Autodesk Inventor part; units mm, degrees
ref_plane "YZ Plane" through (0, 0, 0) normal (1, 0, 0) x (0, 1, 0)
ref_plane "XZ Plane" through (0, 0, 0) normal (0, 1, 0) x (-1, 0, 0)
ref_plane "XY Plane" through (0, 0, 0) normal (0, 0, 1) x (1, 0, 0)
sketch "스케치1" plane through (0, 0, 0) normal (0, 0, 1) x (1, 0, 0)
  circle A0 centre (0, 0) radius 2.5
  dimension "d0" = 5
extrude "돌출1" add sketch "스케치1" along normal mid plane 27
sketch "스케치2" plane through (0, 0, 13.5) normal (0, 0, 1) x (1, 0, 0)
  circle A0 centre (0, 0) radius 5
  dimension "d3" = 10
extrude "돌출2" add sketch "스케치2" along normal blind 3.5
sketch "스케치3" plane through (0, 0, -13.5) normal (0, 0, -1) x (-1, 0, 0)
  circle A0 centre (0, 0) radius 5
  dimension "d6" = 10
extrude "돌출3" add sketch "스케치3" along normal blind 3.5
sketch "스케치4" plane through (0, 0, 0) normal (0, 1, 0) x (-1, 0, 0)
  line L0 (-2, 3) -> (2, 3)
  line L1 (2, 3) -> (2, -3)
  line L2 (2, -3) -> (-2, -3)
  line L3 (-2, -3) -> (-2, 3)
  line L4 (-2, 3) -> (2, -3) construction
  line L5 (2, 3) -> (-2, -3) construction
  point P0 (0, 0)
  dimension "d9" = 4
  dimension "d10" = 6
extrude "돌출4" add sketch "스케치4" along normal mid plane 16
properties part number "15-2"
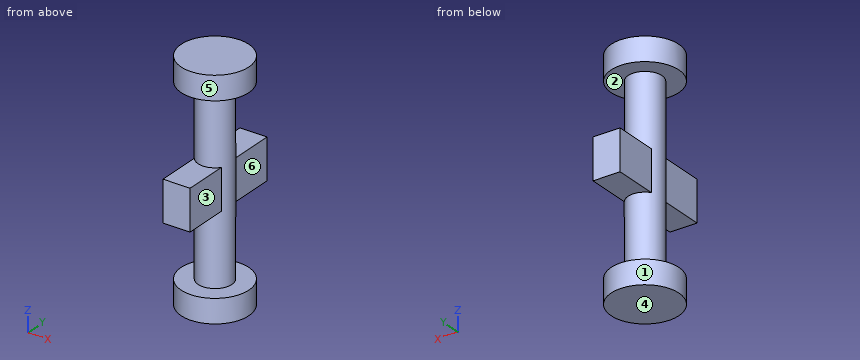
Could you check a few things on this model? Use its own coordinates, in mm. Face numbers are marked on the shaded views. A direction names the side the tool comes from. Give positions to 0.01 mm unless a question says otherwise; leave off trailing zeros. Loops run counter-clockwise (first coordinate to the right, second up) from the corner with the lowest first, then second, coordinate; pieces in that order, holes last. Notation, with made-up numbers: (31, 14.25) -> (75, 14.25) arc R30 cw to (75, 40.25) -> close; hole circle Ø8 at (62.5, -30). An arc over 180 degrees is marked (long way). Return JSON: item names as keys, results as strings.
Item 1: If we section it at C-C on x = 0: List the corners of the cut face in (y, z) for me, plus the area to 3 significant figures.
Geometry results:
{"outline": "(-8, -3) -> (-2.5, -3) -> (-2.5, -13.5) -> (-5, -13.5) -> (-5, -17) -> (5, -17) -> (5, -13.5) -> (2.5, -13.5) -> (2.5, -3) -> (8, -3) -> (8, 3) -> (2.5, 3) -> (2.5, 13.5) -> (5, 13.5) -> (5, 17) -> (-5, 17) -> (-5, 13.5) -> (-2.5, 13.5) -> (-2.5, 3) -> (-8, 3) -> close", "area": "271 mm²"}
Item 2: Which directions (+Z, -Z, +X, -X, +Y, -Y) give clear straight access to the entire face, cutting with the end or side of a thin tool? Please do the marked faces 1, 2 and 3.
Geometry results:
{"face 1": "-Z", "face 2": "none", "face 3": "+X, -Y"}
Item 3: I'm going to push flat-ended pins straight in: pin 1 (2 mm diameter, centred on x = -1.5, z = 8, fed in from -Y); pin 2 (6.5 mm diameter, centred on y = 5, z = -1, fed in from -X); pin 3 (6 mm diameter, centred on y = 0, z = 7, fed in from +X); pin 4 (1.2 mm diameter, centred on x = 0.5, y = 5.5, fed in from -Z). Where does each tip first touch, or does it pass through?
Geometry results:
{"pin 1": "stops at y = -2.45", "pin 2": "stops at x = -2", "pin 3": "stops at x = 2.5", "pin 4": "stops at z = -17"}
Item 4: I need wall thicknesses on L1, parallel to Z at x = 3, y = -3.5; L2, parallel to Z at x = 1.25, y = 2.75; L3, parallel to X at y = 2.25, z = 2. Which ranges of each line are inside material? Lowest first, please. Write a range as from..to.
Geometry results:
{"L1": "z = -17..-13.5, 13.5..17", "L2": "z = -17..-13.5, -3..3, 13.5..17", "L3": "x = -2..2"}
Item 5: If we section it at B-B on y = 4: List the corners of the cut face in (x, z) for me.
Geometry results:
{"outline": "(-3, -17) -> (3, -17) -> (3, -13.5) -> (-3, -13.5) -> close; (-3, 13.5) -> (3, 13.5) -> (3, 17) -> (-3, 17) -> close; (-2, -3) -> (2, -3) -> (2, 3) -> (-2, 3) -> close"}
Item 6: If we section it at D-D on z = 0: List the corners of the cut face in (x, y) for me, plus the area to 3 significant figures.
Geometry results:
{"outline": "(-2, -8) -> (2, -8) -> (2, -1.5) arc R2.5 ccw to (2, 1.5) -> (2, 8) -> (-2, 8) -> (-2, 1.5) arc R2.5 ccw to (-2, -1.5) -> close", "area": "66.0 mm²"}
Item 7: If we section it at A-A on x = -3: List the corners of the cut face in (y, z) for me, plus the area to 3 significant figures.
Geometry results:
{"outline": "(-4, -17) -> (4, -17) -> (4, -13.5) -> (-4, -13.5) -> close; (-4, 13.5) -> (4, 13.5) -> (4, 17) -> (-4, 17) -> close", "area": "56.0 mm²"}
Item 8: We'd pull the mould along Z, two halves only. Please class the marked faces 4, 5 and 6: +Z half, -Z half, draft (parallel to the pull), parting line (faces both ways), or undercut.
Geometry results:
{"face 4": "-Z half", "face 5": "draft", "face 6": "undercut"}
